Check sheet for the modelled part. Datum: model origin and axes. Units: mm. Face numbers are marked on the shaded views. A direction names the side the tool comes from. Coordinates: 2 decimals unless noted, no trailing zeros. Loops run counter-clockwise (first coordinate to the right, second up) from the corner with the lowest first, then second, coordinate; pieces in that order, holes last. Notation, with made-up numbers: (12.5, -11) -> (30.5, -11) arc R17 cw to (30.5, 10) -> close; hole circle Ø9 at (48.25, -19). An arc over 180 degrees is marked (long way). Use one line per item in the form item = value.
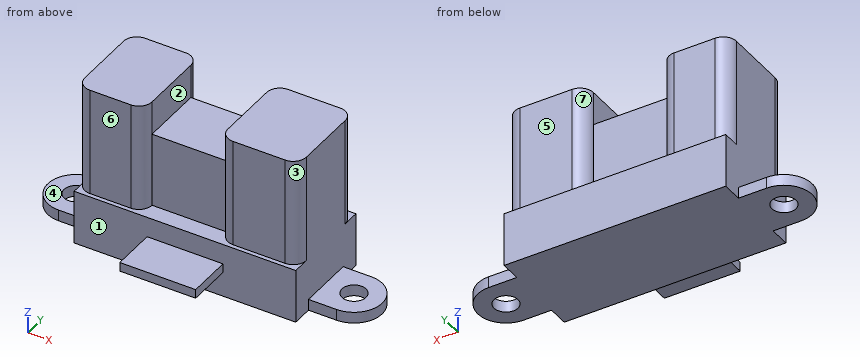
Autodesk Inventor part; units mm, degrees
ref_plane "Work Plane5" through (0, 0, -18.3) normal (0, 0, -1) x (-1, 0, 0)
ref_plane "YZ Plane" through (0, 0, 0) normal (1, 0, 0) x (0, 1, 0)
ref_plane "XZ Plane" through (0, 0, 0) normal (0, 1, 0) x (-1, 0, 0)
sketch "Sketch1" plane through (0, 0, 0) normal (0, 0, 1) x (1, 0, 0)
  line L0 (0, 0) -> (29.5, 0)
  line L1 (29.5, 0) -> (29.5, -18.9)
  line L2 (29.5, -18.9) -> (0, -18.9)
  line L3 (0, -18.9) -> (0, 0)
  dimension "d0" = 29.5
  dimension "d1" = 18.9
extrude "Extrusion1" add sketch "Sketch1" against normal blind 21.6
sketch "Sketch2" plane through (0, 0, 0) normal (0, 0, 1) x (1, 0, 0)
  line L0 (0, 0) -> (29.5, 0)
  line L1 (29.5, -18.9) -> (0, -18.9)
  line L2 (0, -18.9) -> (0, 0)
  line L3 (0, 0) -> (29.5, 0)
  line L4 (29.5, 0) -> (29.5, -13)
  line L5 (29.5, -13) -> (0, -13)
  line L6 (0, -13) -> (0, 0)
  line L7 (9.7099, -18.9) -> (19.8099, -18.9)
  line L8 (19.8099, -18.9) -> (19.8099, -13)
  line L9 (19.8099, -13) -> (9.7099, -13)
  line L10 (9.7099, -13) -> (9.7099, -18.9)
  line L11 (29.5, 0) -> (29.5, -18.9)
  dimension "d6" = 13
  dimension "d11" = 10.1
  dimension "d39" = 9.6901
extrude "Extrusion2" cut sketch "Sketch2" against normal blind 21.6 contours L5 L10 L1 L2 | L11 L1 L8 L5
sketch "Sketch4" plane through (0, 0, 0) normal (0, 0, 1) x (1, 0, 0)
  line L0 (9.7099, -13) -> (9.7099, -18.9)
  line L1 (29.5, -18.9) -> (0, -18.9)
  line L2 (19.8099, -18.9) -> (19.8099, -13)
  line L3 (19.8099, -13) -> (29.5, -13)
  line L4 (29.5, 0) -> (29.5, -18.9)
  line L5 (0, 0) -> (29.5, 0)
  line L6 (0, -18.9) -> (0, 0)
  line L7 (0, -13) -> (9.7099, -13)
extrude "Extrusion3" cut sketch "Sketch4" against normal blind 14.4 contours L7 L6 L5 L4 L3 L2 L1 L0
sketch "Sketch5" plane through (0, 0, -14.4) normal (0, 0, 1) x (1, 0, 0)
  line L0 (29.5, 0) -> (29.5, -13)
  line L1 (0, 0) -> (29.5, 0)
  line L2 (0, -13) -> (0, 0)
  line L3 (0, -0.5461) -> (8.95, -0.5461)
  line L4 (8.95, -0.5461) -> (8.95, -12.4461)
  line L5 (8.95, -12.4461) -> (0, -12.4461)
  line L6 (0, -12.4461) -> (0, -0.5461)
  line L7 (19.05, -0.5461) -> (29.5, -0.5461)
  line L8 (29.5, -0.5461) -> (29.5, -12.4461)
  line L9 (29.5, -12.4461) -> (19.05, -12.4461)
  line L10 (19.05, -12.4461) -> (19.05, -0.5461)
  point P0 (33.25, -13)
  dimension "d22" = 8.95
  dimension "d23" = 10.45
  dimension "d24" = 11.9
  dimension "d25" = 11.9
  dimension "d26" = 0.5461
  dimension "d27" = 0.5461
extrude "Extrusion4" add sketch "Sketch5" along normal blind 14.4
fillet "Fillet1" radius 1.75 8 edges at (8.95, -0.5461, -7.2) (8.95, -12.4461, -7.2) (0, -0.5461, -7.2) (29.5, -0.5461, -7.2) (19.05, -0.5461, -7.2) (29.5, -12.4461, -7.2) (0, -12.4461, -7.2) (19.05, -12.4461, -7.2)
sketch "Sketch6" plane through (0, 0, -14.4) normal (0, 0, 1) x (1, 0, 0)
  line L0 (19.05, -10.6961) -> (19.05, -2.2961)
  line L1 (0, 0) -> (29.5, 0)
  line L2 (8.95, -2.2961) -> (8.95, -10.6961)
  line L3 (8.95, -2.2987) -> (19.05, -2.2987)
  line L4 (19.05, -2.2987) -> (19.05, -10.6987)
  line L5 (19.05, -10.6987) -> (8.95, -10.6987)
  line L6 (8.95, -10.6987) -> (8.95, -2.2987)
  dimension "d31" = 8.4
  dimension "d32" = 2.2987
extrude "Extrusion5" add sketch "Sketch6" along normal blind 9.9
sketch "Sketch8" plane through (0, 0, -21.6) normal (0, 0, -1) x (-1, 0, 0)
  line L0 (-9.7099, -18.9) -> (-9.7099, -13)
  line L1 (-9.7099, -13) -> (0, -13)
  line L2 (0, -13) -> (0, 0)
  line L3 (0, 0) -> (-29.5, 0)
  line L4 (-29.5, 0) -> (-29.5, -13)
  line L5 (-29.5, -13) -> (-19.8099, -13)
  line L6 (-19.8099, -13) -> (-19.8099, -18.9)
  line L7 (-19.8099, -18.9) -> (-9.7099, -18.9)
  circle A0 centre (-33.25, -6.5) radius 3.75
  circle A1 centre (-33.25, -6.5) radius 1.6
  circle A2 centre (3.75, -6.5) radius 3.75
  circle A3 centre (3.75, -6.5) radius 1.6
  line L8 (-33.25, -2.75) -> (-29.5, -2.75)
  line L9 (-33.25, -10.25) -> (-29.5, -10.25)
  line L10 (3.75, -10.25) -> (0, -10.25)
  line L11 (3.75, -2.75) -> (0, -2.75)
  dimension "d40" = 37
  dimension "d41" = 7.5
  dimension "d42" = 3.2
  dimension "d43" = 7.5
  dimension "d44" = 3.2
  dimension "d46" = 29.5
extrude "Extrusion6" add sketch "Sketch8" against normal blind 1.5 contours L2 A2 L10 | L2 L11 A2 | A2 | L9 A0 L4 | A0 L8 L4 | A0
sketch "Sketch10" plane through (0, 0, -14.4) normal (0, 0, 1) x (1, 0, 0)
  line L0 (9.7099, -18.9) -> (9.7099, -13)
  line L1 (9.7099, -13) -> (19.8099, -13)
  line L2 (19.8099, -13) -> (19.8099, -18.9)
  line L3 (19.8099, -18.9) -> (9.7099, -18.9)
  line L4 (9.7099, -18.9) -> (9.7099, -13)
  point P0 (0, 0)
extrude "Extrusion7" cut sketch "Sketch10" against normal blind 6
ref_plane "Work Plane5" through (0, 0, -18.3) normal (0, 0, -1) x (-1, 0, 0)
sketch "Sketch11" plane through (0, 0, -18.3) normal (0, 0, -1) x (-1, 0, 0)
  line L0 (-19.8099, -18.9) -> (-9.7099, -18.9)
  line L1 (-9.7099, -13) -> (-19.8099, -13)
  line L2 (-19.8099, -13) -> (-19.8099, -18.9)
  line L3 (-19.8099, -18.9) -> (-9.7099, -18.9)
  line L4 (-9.7099, -18.9) -> (-9.7099, -13)
  point P0 (0, 0)
extrude "Extrusion8" add sketch "Sketch11" against normal blind 1.2
sketch "Sketch12" plane through (0, 0, -20.4) normal (0, 0, 1) x (1, 0, 0)
  line L0 (9.7099, -13) -> (0, -13)
  line L1 (19.8099, -13) -> (19.8099, -18.9)
  line L2 (9.7099, -13) -> (19.8099, -13)
  line L3 (19.8099, -13) -> (19.8099, -18.9)
  line L4 (19.8099, -18.9) -> (9.7099, -18.9)
  line L5 (9.7099, -18.9) -> (9.7099, -13)
  point P0 (0, 0)
extrude "Extrusion9" cut sketch "Sketch12" against normal blind 1.2
properties part number "Sharp 2Y0A02"
(1) Mould release check, pull along X, two halves, no side actions. Record for the marked faces 1, 2 and 3: +X half, -X half, draft (parallel to the pull), parting line (faces both ways), or undercut.
Established:
face_1 = draft
face_2 = undercut
face_3 = +X half
(2) Section check C-C, the plane x = 24. Record the boundary of the cut face in (y, z).
Established:
outline = (-13, -21.6) -> (0, -21.6) -> (0, -14.4) -> (-0.55, -14.4) -> (-0.55, 0) -> (-12.45, 0) -> (-12.45, -14.4) -> (-13, -14.4) -> close
(3) Tool access check on the marked faces 4, 5, 6 and 7. Record the directions out of +Z, -Z, +X, -X, +Y, -Y that give a thin tool (end or side, any length) a straight path to the whole face; none if there is none.
Established:
face_4 = +Z, -X, +Y, -Y
face_5 = +Z, +X, -X, +Y
face_6 = +Z, +X, -X, -Y
face_7 = +Z, +Y
(4) Go/stop test with flat-tipped pins: P1, Ø1, axis at y = -17, z = -18, coming from the +X side; P2, Ø8, axis at x = 12.5, z = -7, coming from the +Y side; P3, Ø1.3, axis at y = -16.5, z = -18, coming from the -X side. Record where each tip stops, or that it passes through.
Established:
P1 = 19.81
P2 = -1.12
P3 = 9.71
(5) Scan lines: line 1 along Y through (x, z) = (33.25, -20.65); line 2 along Z through (x, y) = (16.5, -14.5); line 3 along Z through (x, y) = (16, -8.75). Record each from-to range of solid material in increasing order.
Established:
line_1 = -10.25 to -8.1, -4.9 to -2.75
line_2 = -18.3 to -17.1
line_3 = -21.6 to -4.5
(6) Section check A-A, the plane y = -6.5. Record the boundary of the cut face in (x, z), plus the area to 3 significant figures.
Established:
outline = (-7.5, -21.6) -> (-5.35, -21.6) -> (-5.35, -20.1) -> (-7.5, -20.1) -> close; (-2.15, -21.6) -> (31.65, -21.6) -> (31.65, -20.1) -> (29.5, -20.1) -> (29.5, 0) -> (19.05, 0) -> (19.05, -4.5) -> (8.95, -4.5) -> (8.95, 0) -> (0, 0) -> (0, -20.1) -> (-2.15, -20.1) -> close; (34.85, -21.6) -> (37, -21.6) -> (37, -20.1) -> (34.85, -20.1) -> close
area = 605 mm²
(7) Section check D-D, the plane y = -9.5. Record the boundary of the cut face in (x, z).
Established:
outline = (-6, -21.6) -> (35.5, -21.6) -> (35.5, -20.1) -> (29.5, -20.1) -> (29.5, 0) -> (19.05, 0) -> (19.05, -4.5) -> (8.95, -4.5) -> (8.95, 0) -> (0, 0) -> (0, -20.1) -> (-6, -20.1) -> close
